The drawing under review shows one solid part. Ordinate dimensions are in mm from its lowest x, y, z. Give positions to 0.01 mm unless a question says otherwise; leave off trailing zeros. Write each loop counter-clockwise with the first axis right and the second up, starting at its lowest first coordinate (ties: lowest second). Pieces come first, ordered by that corner, then holes. Notation, with made-up numbers: M 86.25,80.5 L 130.25,80.5 A15 ccw 130.25,85.5 Z; hole C 0,-15.75 d10. An arc over 180 degrees is marked long. Use one line per item in the form item = value. Start each with the question number.
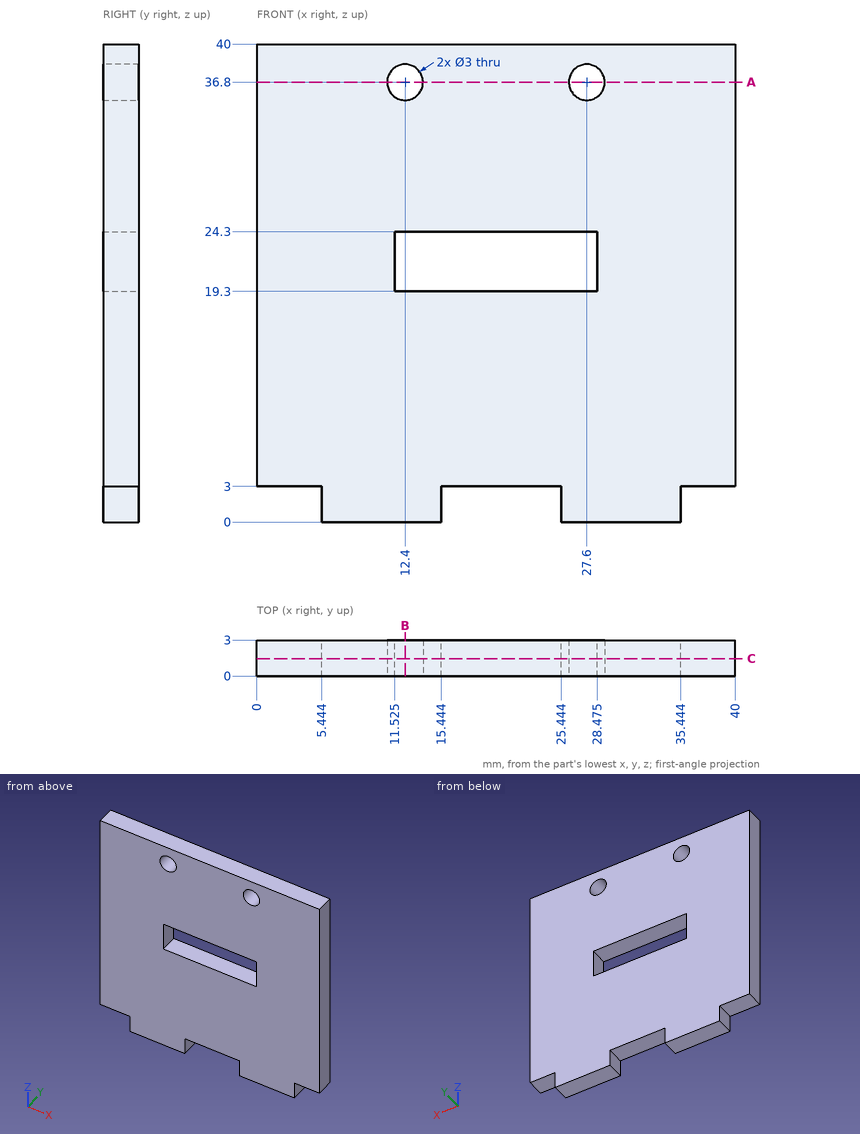
1. We need section C-C (y = 1.45). State the section outline as (x, z) points (1 decimal).
2. Clearance check with flat-ended pins moving along their axes: pin 1 Ø1.5 at (y, z) = (2, 1.5) entering from -X (1 decimal); pin 2 Ø5 at (x, z) = (12.4, 36.8) entering from -Y; pin 3 Ø0.9 at (y, z) = (1, 1) entering from +X (1 decimal); pin 4 Ø0.9 at (x, y) = (2, 1.5) entering from -Z. State where each tip first meets the part, or that it passes through.
3. We need section A-A (z = 36.8). State the section outline as (x, y) points, and give its area (3 significant figures).
4. To check wall thickness, follow L1, parallel to X at y = 1.25, z = 36.8; L2, parallel to Z at x = 13.5, y = 2.85; L3, parallel to Z at x = 14.5, y = 0.4. State the ranges of each line that lie inside material, in increasing order.
5. We need section B-B (x = 12.4). State the section outline as (y, z) points.
Answer block:
q1.outline = M 0,3 L 5.4,3 L 5.4,0 L 15.4,0 L 15.4,3 L 25.4,3 L 25.4,0 L 35.4,0 L 35.4,3 L 40,3 L 40,40 L 0,40 Z; hole C 12.4,36.8 d3; hole M 11.5,19.3 L 28.5,19.3 L 28.5,24.3 L 11.5,24.3 Z; hole C 27.6,36.8 d3
q2.pin_1 = 5.4
q2.pin_2 = 0
q2.pin_3 = 35.4
q2.pin_4 = 3
q3.outline = M 0,0 L 10.9,0 L 10.9,3 L 0,3 Z; M 13.9,0 L 26.1,0 L 26.1,3 L 13.9,3 Z; M 29.1,0 L 40,0 L 40,3 L 29.1,3 Z
q3.area = 102 mm^2
q4.L1 = 0 to 10.9, 13.9 to 26.1, 29.1 to 40
q4.L2 = 0 to 19.3, 24.3 to 35.78, 37.82 to 40
q4.L3 = 0 to 19.3, 24.3 to 40
q5.outline = M 0,0 L 3,0 L 3,19.3 L 0,19.3 Z; M 0,24.3 L 3,24.3 L 3,35.3 L 0,35.3 Z; M 0,38.3 L 3,38.3 L 3,40 L 0,40 Z
